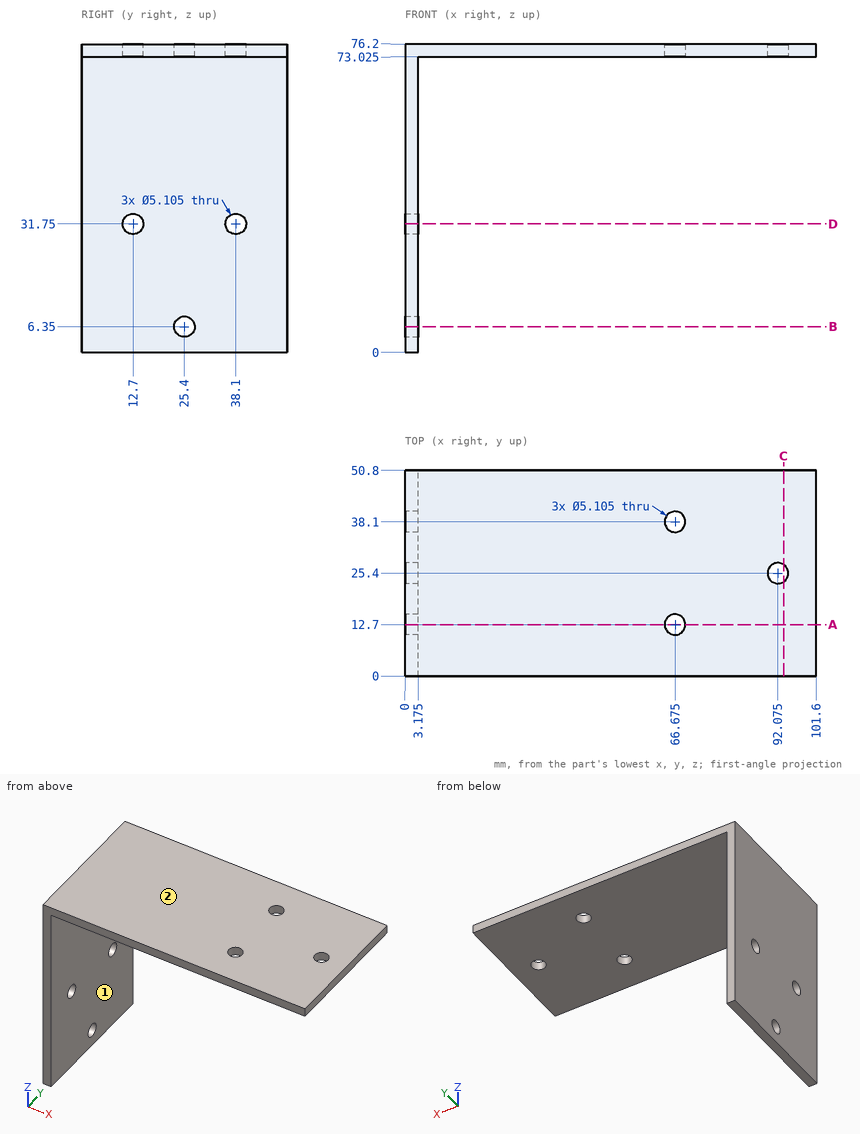
Could you check a few things on this drawing? It's one solid part, dimensions in mm from its lowest x, y, z. A direction names the side the tool comes from. Coordinates: 2 decimals unless noted, no trailing zeros. Order: outer loops, then holes, each group sorted by start corner. A loop starts at its lowest first (then second) coordinate and runs counter-clockwise, first axis right, second up.
1) Imagine slicing it at A-A on y = 12.7. List the corners of the cut face in (x, z) for me (1 decimal).
2) I need wall thicknesses on line 1 (Z direction, x = 1, y = 38); line 2 (X direction, y = 45, z = 11) (1 decimal); line 3 (Z direction, x = 35.5, y = 10.5) (1 decimal). Which ranges of each line are inside material? Lowest first, please.
3) Imagine slicing it at D-D on z = 31.75. List the corners of the cut face in (x, y) for me (1 decimal).
4) Which directions (+Z, -Z, +X, -X, +Y, -Y) give clear straight access to the entire face, cutting with the end or side of a thin tool? Please do the marked faces 1 and 2.
5) Will these pins go through, and if not, where does the flat tip stop? pin 1 (10 mm diameter, centred on x = 42, y = 25.5, fed in from -Z) (3 decimals); pin 2 (10 mm diameter, centred on y = 13.5, z = 29, fed in from +X) (3 decimals); pin 3 (4.5 mm diameter, centred on x = 66.675, y = 12.7, fed in from +Z).
6) Imagine slicing it at B-B on z = 6.35. List the corners of the cut face in (x, y) for me (1 decimal), and give its area (3 significant figures).
7) Imagine slicing it at C-C on x = 93.5. List the corners of the cut face in (y, z) for me (1 decimal), and give its area (3 significant figures).
Response values:
1. outline: (0, 0) - (3.2, 0) - (3.2, 29.2) - (0, 29.2) - close; (0, 34.3) - (3.2, 34.3) - (3.2, 73) - (64.1, 73) - (64.1, 76.2) - (0, 76.2) - close; (69.2, 73) - (101.6, 73) - (101.6, 76.2) - (69.2, 76.2) - close
2. line 1: z = 0 to 29.2, 34.3 to 76.2
2. line 2: x = 0 to 3.2
2. line 3: z = 73 to 76.2
3. outline: (0, 0) - (3.2, 0) - (3.2, 10.1) - (0, 10.1) - close; (0, 15.3) - (3.2, 15.3) - (3.2, 35.5) - (0, 35.5) - close; (0, 40.7) - (3.2, 40.7) - (3.2, 50.8) - (0, 50.8) - close
4. face 1: -Z, +X, +Y, -Y
4. face 2: +Z, +X, -X, +Y, -Y
5. pin 1: stops at z = 73.025
5. pin 2: stops at x = 3.175
5. pin 3: passes through
6. outline: (0, 0) - (3.2, 0) - (3.2, 22.8) - (0, 22.8) - close; (0, 28) - (3.2, 28) - (3.2, 50.8) - (0, 50.8) - close
6. area: 145 mm2
7. outline: (0, 73) - (23.3, 73) - (23.3, 76.2) - (0, 76.2) - close; (27.5, 73) - (50.8, 73) - (50.8, 76.2) - (27.5, 76.2) - close
7. area: 148 mm2
